Autodesk Inventor part; units mm, degrees
ref_plane "YZ Plane" through (0, 0, 0) normal (1, 0, 0) x (0, 1, 0)
ref_plane "XZ Plane" through (0, 0, 0) normal (0, 1, 0) x (-1, 0, 0)
ref_plane "XY Plane" through (0, 0, 0) normal (0, 0, 1) x (1, 0, 0)
sketch "Sketch2" plane through (0, 0, 0) normal (0, 0, 1) x (1, 0, 0)
  arc A0 (-52, -72) -> (-47, -77) centre (-47, -72) ccw
  line L0 (-52, 72) -> (-52, -72)
  arc A1 (-47, 77) -> (-52, 72) centre (-47, 72) ccw
  line L1 (47, 77) -> (-47, 77)
  arc A2 (52, 72) -> (47, 77) centre (47, 72) ccw
  line L2 (52, -72) -> (52, 72)
  arc A3 (47, -77) -> (52, -72) centre (47, -72) ccw
  line L3 (-47, -77) -> (47, -77)
  circle A4 centre (44.5, -69.5) radius 1.65
  circle A5 centre (-44.5, -69.5) radius 1.65
  circle A6 centre (-44.5, 69.5) radius 1.65
  circle A7 centre (44.5, 69.5) radius 1.65
  point P0 (0, 0)
extrude "Extrusion2" add sketch "Sketch2" along normal blind 3
sketch "Sketch3" plane through (0, 0, 0) normal (0, 0, -1) x (-1, 0, 0)
  arc A0 (-50, 61) -> (-36, 75) centre (-50, 75) ccw
  line L0 (36, 75) -> (-36, 75)
  arc A1 (36, 75) -> (50, 61) centre (50, 75) ccw
  line L1 (50, -61) -> (50, 61)
  line L2 (-50, 61) -> (-50, -61)
  arc A2 (-36, -75) -> (-50, -61) centre (-50, -75) ccw
  line L3 (-36, -75) -> (36, -75)
  arc A3 (50, -61) -> (36, -75) centre (50, -75) ccw
  arc A4 (-49.8, 60.8014) -> (-35.8014, 74.8) centre (-50, 75) ccw
  line L4 (-49.8, 60.8014) -> (-49.8, -60.8014)
  arc A5 (-35.8014, -74.8) -> (-49.8, -60.8014) centre (-50, -75) ccw
  line L5 (-35.8014, -74.8) -> (35.8014, -74.8)
  arc A6 (49.8, -60.8014) -> (35.8014, -74.8) centre (50, -75) ccw
  line L6 (49.8, -60.8014) -> (49.8, 60.8014)
  arc A7 (35.8014, 74.8) -> (49.8, 60.8014) centre (50, 75) ccw
  line L7 (35.8014, 74.8) -> (-35.8014, 74.8)
  arc A8 (-47.8, 58.9501) -> (-33.9501, 72.8) centre (-50, 75) ccw
  line L8 (-47.8, 58.9501) -> (-47.8, -58.9501)
  arc A9 (-33.9501, -72.8) -> (-47.8, -58.9501) centre (-50, -75) ccw
  line L9 (-33.9501, -72.8) -> (33.9501, -72.8)
  arc A10 (47.8, -58.9501) -> (33.9501, -72.8) centre (50, -75) ccw
  line L10 (47.8, -58.9501) -> (47.8, 58.9501)
  arc A11 (33.9501, 72.8) -> (47.8, 58.9501) centre (50, 75) ccw
  line L11 (33.9501, 72.8) -> (-33.9501, 72.8)
  point P0 (0, 0)
  dimension "d4" = 0.2
  dimension "d5" = 2
extrude "Extrusion3" add sketch "Sketch3" along normal blind 2 contours A4 L7 A7 L6 A6 L5 A5 L4
sketch "Sketch4" plane through (0, 0, 3) normal (0, 0, 1) x (1, 0, 0)
  line L0 (11.65, 34.65) -> (11.65, -34.65)
  arc A0 (11.65, 34.65) -> (10.65, 35.65) centre (10.65, 34.65) ccw
  line L1 (-11.65, 35.65) -> (10.65, 35.65)
  arc A1 (-11.65, 35.65) -> (-12.65, 34.65) centre (-11.65, 34.65) ccw
  line L2 (-12.65, -34.65) -> (-12.65, 34.65)
  arc A2 (-12.65, -34.65) -> (-11.65, -35.65) centre (-11.65, -34.65) ccw
  line L3 (10.65, -35.65) -> (-11.65, -35.65)
  arc A3 (10.65, -35.65) -> (11.65, -34.65) centre (10.65, -34.65) ccw
  line L4 (11.95, -34.65) -> (11.95, 34.65)
  arc A4 (11.95, 34.65) -> (10.65, 35.95) centre (10.65, 34.65) ccw
  line L5 (10.65, 35.95) -> (-11.65, 35.95)
  arc A5 (-11.65, 35.95) -> (-12.95, 34.65) centre (-11.65, 34.65) ccw
  line L6 (-12.95, 34.65) -> (-12.95, -34.65)
  arc A6 (-12.95, -34.65) -> (-11.65, -35.95) centre (-11.65, -34.65) ccw
  line L7 (-11.65, -35.95) -> (10.65, -35.95)
  arc A7 (10.65, -35.95) -> (11.95, -34.65) centre (10.65, -34.65) ccw
  point P0 (0, 0)
  dimension "d10" = 0.3
extrude "Extrusion4" cut sketch "Sketch4" against normal up to surface (3 mm away) contours L0 A3 L3 A2 L2 A1 L1 A0 | A7 L7 A6 L6 A5 L5 A4 L4
sketch "Sketch5" plane through (0, 0, 0) normal (0, 0, -1) x (-1, 0, 0)
  circle A0 centre (15.5, 37.5) radius 1.5
  circle A1 centre (-15.5, 37.5) radius 1.5
  circle A2 centre (15.5, -37.5) radius 1.5
  circle A3 centre (-15.5, -37.5) radius 1.5
  circle A4 centre (15.5, -37.5) radius 1.7
  circle A5 centre (15.5, 37.5) radius 1.7
  circle A6 centre (-15.5, 37.5) radius 1.7
  circle A7 centre (-15.5, -37.5) radius 1.7
  point P0 (0, 0)
  dimension "d11" = 0.2
  dimension "d12" = 0.2
  dimension "d13" = 0.2
  dimension "d14" = 0.2
extrude "Extrusion5" cut sketch "Sketch5" against normal up to surface (3 mm away) contours A0 | A1 | A2 | A3 | A4 | A5 | A6 | A7
sketch "Sketch6" plane through (0, 0, 3) normal (0, 0, 1) x (1, 0, 0)
  line L0 (-25.9, 6.1) -> (-38.1, 6.1)
  line L1 (-38.1, 6.1) -> (-38.1, -6.1)
  line L2 (-38.1, -6.1) -> (-25.9, -6.1)
  line L3 (-25.9, -6.1) -> (-25.9, 6.1)
  line L4 (-25.9, 6.1) -> (-38.1, -6.1) construction
  line L5 (-38.1, 6.1) -> (-25.9, -6.1) construction
  line L6 (-52, 72) -> (-52, -72)
  line L7 (47, 77) -> (-47, 77)
  line L8 (52, -72) -> (52, 72)
  line L9 (52, 0) -> (-52, 0)
  point P0 (0, 0)
  point P1 (-32, 0)
  dimension "d17" = 12.2
  dimension "d18" = 12.2
  dimension "d19" = 20
extrude "Extrusion6" cut sketch "Sketch6" against normal up to surface (3 mm away)
pattern_linear "Rectangular Pattern1" count 3 spacing 20 along (0, -1, 0) count 3 spacing 20 along (0, 1, 0) of "Extrusion6"
sketch "Sketch9" plane through (0, 0, 0) normal (0, 0, -1) x (-1, 0, 0)
  line L0 (-13.95, -31.8) -> (-18.95, -31.8)
  line L1 (-18.95, -31.8) -> (-18.95, 31.8)
  line L2 (-18.95, 31.8) -> (-13.95, 31.8)
  line L3 (-13.95, 31.8) -> (-13.95, -31.8)
  circle A0 centre (-15.5, -37.5) radius 1.7
  circle A1 centre (-15.5, 37.5) radius 1.7
  line L4 (-11.95, -34.65) -> (-11.95, 34.65)
  point P0 (0, 0)
  dimension "d38" = 4
  dimension "d40" = 4
  dimension "d41" = 2
  dimension "d42" = 5
extrude "Extrusion9" add sketch "Sketch9" along normal blind 4 contours L0 L1 L2 L3
sketch "Sketch10" plane through (0, 0, 0) normal (0, 0, -1) x (-1, 0, 0)
  point P0 (0, 0)
sketch "Sketch11" plane through (0, 0, 0) normal (0, 0, -1) x (-1, 0, 0)
  line L0 (25.9, 33.9) -> (38.1, 33.9)
  line L1 (38.1, 33.9) -> (40.1, 33.9)
  line L2 (40.1, 33.9) -> (40.1, 46.1)
  line L3 (40.1, 46.1) -> (38.1, 46.1)
  line L4 (38.1, 46.1) -> (38.1, 33.9)
  line L5 (25.9, 46.1) -> (25.9, 33.9)
  line L6 (25.9, 46.1) -> (23.9, 46.1)
  line L7 (23.9, 46.1) -> (23.9, 33.9)
  line L8 (23.9, 33.9) -> (25.9, 33.9)
  line L9 (25.9, 33.9) -> (25.9, 46.1)
  point P0 (0, 0)
  dimension "d45" = 2
  dimension "d46" = 2
extrude "Extrusion10" add sketch "Sketch11" along normal up to surface (2 mm away)
pattern_linear "Rectangular Pattern3" count 5 spacing 20 along (0, -1, 0) of "Extrusion10"
equation "\"d46\" = d45"
properties part number "lid"
Geometry check sheet. Reference: the model listing, model coordinates, mm. A direction names the side the tool comes from. Coordinates: 2 decimals unless noted, no trailing zeros. Order: outer loops, then holes, each group sorted by start corner. A loop starts at its lowest first (then second) coordinate and runs counter-clockwise, first axis right, second up. Notation, with made-up numbers: (-13.5, -21) - (0.5, -21) arc R23 ccw to (0.5, -6) - close; hole circle Ø4 at (-25.5, -3.75). An arc over 180 degrees is marked (long way). Answer as a JSON object with one key per item and string values. Group by question number.
Item 1: Depth check by flat-ended pin: pin 1 Ø1 at (y, z) = (-43, -1.5) entering from -X; pin 2 Ø1 at (x, y) = (-39, -39) entering from -Z; pin 3 Ø1.5 at (x, z) = (-39, -1) entering from -Y. Enter the tip coordinate at first touch or a pass-through.
Item 2: Sectioned sample at B-B, the plane x = 15.5. Record the cut outline in (y, z), and give its area (3 significant figures).
Item 3: Sectioned sample at C-C, the plane y = 37.5. Record the cut outline in (x, z).
Item 4: Draft check along Y on faces 3 (the face through (52, -1, 1)), 4 (the face through (-32, -13.9, 2)), 5 (the face through (-38.65, 63.44, -0.99)), 6 (the face through (51, -75, 1)). Enter one of: +Y half, -Y half, draft (parallel to the pull), parting line (faces both ways), or undercut.
Item 5: Sectioned sample at D-D, the plane y = -4.5. Record the cut outline in (x, z), and give its area (3 significant figures).
Item 6: Tool access check on faces 1 (the face through (-38.1, 20, 1)), 2 (the face through (16, 31.8, -2)). Record the directions out of +Z, -Z, +X, -X, +Y, -Y that give a thin tool (end or side, any length) a straight path to the whole face; none if there is none.
Item 7: Sectioned sample at A-A, the plane x = -4. Record the cut outline in (y, z), and give its area (3 significant figures).
Item 8: Scan lines: probe 1 along Y at (x, z) = (44.5, 1.1); probe 2 along X at (y, z) = (-45.5, -0.25); probe 3 along X at (y, z) = (3, -1). Record each from-to range of solid material in increasing order.
Resolved:
{
 "1": {"pin 1": "x = -49.8", "pin 2": "z = -2", "pin 3": "y = -67.03"},
 "2": {"outline": "(-77, 0) - (-74.8, 0) - (-74.8, -2) - (-72.8, -2) - (-72.8, 0) - (-39.2, 0) - (-39.2, 3) - (-77, 3) - close; (-35.8, 0) - (-31.8, 0) - (-31.8, -4) - (31.8, -4) - (31.8, 0) - (35.8, 0) - (35.8, 3) - (-35.8, 3) - close; (39.2, 0) - (72.8, 0) - (72.8, -2) - (74.8, -2) - (74.8, 0) - (77, 0) - (77, 3) - (39.2, 3) - close", "area": "704 mm^2"},
 "3": {"outline": "(-52, 0) - (-49.8, 0) - (-49.8, -2) - (-47.8, -2) - (-47.8, 0) - (-40.1, 0) - (-40.1, -2) - (-38.1, -2) - (-38.1, 3) - (-52, 3) - close; (-25.9, -2) - (-23.9, -2) - (-23.9, 0) - (-17.2, 0) - (-17.2, 3) - (-25.9, 3) - close; (-13.8, 0) - (13.8, 0) - (13.8, 3) - (-13.8, 3) - close; (17.2, 0) - (47.8, 0) - (47.8, -2) - (49.8, -2) - (49.8, 0) - (52, 0) - (52, 3) - (17.2, 3) - close"},
 "4": {"face 3": "draft", "face 4": "undercut", "face 5": "undercut", "face 6": "-Y half"},
 "5": {"outline": "(-52, 0) - (-49.8, 0) - (-49.8, -2) - (-47.8, -2) - (-47.8, 0) - (-40.1, 0) - (-40.1, -2) - (-38.1, -2) - (-38.1, 3) - (-52, 3) - close; (-25.9, -2) - (-23.9, -2) - (-23.9, 0) - (-12.95, 0) - (-12.95, 3) - (-25.9, 3) - close; (11.95, 0) - (13.95, 0) - (13.95, -4) - (18.95, -4) - (18.95, 0) - (47.8, 0) - (47.8, -2) - (49.8, -2) - (49.8, 0) - (52, 0) - (52, 3) - (11.95, 3) - close", "area": "237 mm^2"},
 "6": {"face 1": "+Z, -Z", "face 2": "-Z"},
 "7": {"outline": "(-77, 0) - (-74.8, 0) - (-74.8, -2) - (-72.8, -2) - (-72.8, 0) - (-35.95, 0) - (-35.95, 3) - (-77, 3) - close; (35.95, 0) - (72.8, 0) - (72.8, -2) - (74.8, -2) - (74.8, 0) - (77, 0) - (77, 3) - (35.95, 3) - close", "area": "254 mm^2"},
 "8": {"probe 1": "-77 to -71.15, -67.85 to 67.85, 71.15 to 77", "probe 2": "-49.8 to -47.8, -40.1 to -38.1, -25.9 to -23.9, 47.8 to 49.8", "probe 3": "-49.8 to -47.8, -40.1 to -38.1, -25.9 to -23.9, 13.95 to 18.95, 47.8 to 49.8"}
}
